from build123d import *

# Parameters (mm, degrees)
SKETCH1_W           = 76.2
SKETCH1_H           = 152.4
BOSS_EXTRUDE1_DEPTH = 3.175
SKETCH2_R           = 4.4196
CUT_EXTRUDE1_DEPTH  = 86.430512699
CUT_EXTRUDE2_DEPTH  = 86.430512699
FILLET1_R           = 12.7


with BuildPart() as part:
    # Sketch1 → Boss-Extrude1 (new, symmetric)
    with BuildSketch(Plane(origin=(0, 0, 0), x_dir=(1, 0, 0), z_dir=(0, 1, 0))):
        Rectangle(SKETCH1_W, SKETCH1_H)
    extrude(amount=BOSS_EXTRUDE1_DEPTH, both=True)

    # Sketch2 → Cut-Extrude1 (cut, through all)
    with BuildSketch(Plane(origin=(0, 3.175, 0), x_dir=(1, 0, 0), z_dir=(0, 1, 0))):
        with Locations(Location((-19.05, 57.15, 0), (0, 0, 270))):
            Circle(SKETCH2_R)
        with Locations(Location((19.05, 57.15, 0), (0, 0, 270))):
            Circle(SKETCH2_R)
        with Locations(Location((19.05, 19.05, 0), (0, 0, 270))):
            Circle(SKETCH2_R)
        with Locations(Location((19.05, -19.05, 0), (0, 0, 270))):
            Circle(SKETCH2_R)
        with Locations(Location((19.05, -57.15, 0), (0, 0, 270))):
            Circle(SKETCH2_R)
        with Locations(Location((-19.05, 19.05, 0), (0, 0, 270))):
            Circle(SKETCH2_R)
        with Locations(Location((-19.05, -19.05, 0), (0, 0, 270))):
            Circle(SKETCH2_R)
        with Locations(Location((-19.05, -57.15, 0), (0, 0, 270))):
            Circle(SKETCH2_R)
    extrude(amount=-CUT_EXTRUDE1_DEPTH, mode=Mode.SUBTRACT)

    # Sketch3 → Cut-Extrude2 (cut, through all)
    with BuildSketch(Plane(origin=(0, 3.175, 0), x_dir=(1, 0, 0), z_dir=(0, 1, 0))):
        Polygon((-38.1, 51.055282861), (-12.955282861, 76.2), (-38.1, 76.2), align=None)
        Polygon((12.955282861, 76.2), (38.1, 76.2), (38.1, 51.055282861), align=None)
    extrude(amount=-CUT_EXTRUDE2_DEPTH, mode=Mode.SUBTRACT)

    # Fillet1
    fillet1_edges = [part.edges().sort_by_distance(p)[0] for p in [
        (-38.1, 0, -51.055282861),
        (-12.955282861, 0, -76.2),
        (38.1, 0, -51.055282861),
        (12.955282861, 0, -76.2),
        (38.1, 0, 76.2),
        (-38.1, 0, 76.2),
    ]]
    fillet(fillet1_edges, radius=FILLET1_R)


solid = part.part
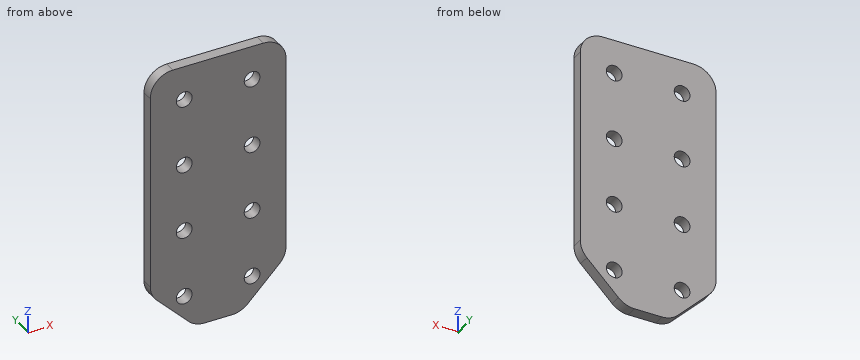
Input: part model. Units: mm. Frame: model coordinates. Give positions to 0.01 mm unless a question says otherwise; leave off trailing zeros. Loops run counter-clockwise (first coordinate to the right, second up) from the corner with the lowest first, then second, coordinate; pieces in that order, holes last. Notation, with made-up numbers: (59.5, 28) -> (76.5, 28) arc R32 ccw to (76.5, 56) -> close; hole circle Ø10 at (66, 57). An arc over 180 degrees is marked (long way). Answer as a JSON object with one key per item and string values. Group by question number.
Item 1: Cut plane B-B, the plane z = -19.05. Return the cut outline in (x, y) (3 decimals).
Item 2: Pin query (flat end, axial travel): P1, Ø14, axis at x = 19.05, z = -19.05, coming from the +Y side (3 decimals). Return the tip coordinate at first contact, or that it passes through.
Item 3: Cut plane C-C, the plane z = -57.15. Return the cut outline in (x, y) (3 decimals), and give its area (3 significant figures).
Item 4: Cut plane A-A, the plane y = -1.75. State how many separate pieces and enclosed holes the cut face has, and give its area (3 significant figures).
Item 5: Line query: probe 1 along X at (y, z) = (0.25, -19.05); probe 2 along Z at (x, y) = (19.5, -2.5); probe 3 along X at (y, z) = (-1, 56.5). Output: solid intervals per line, ascending.
Item 6: Cut plane D-D, the plane x = 28. Return the cut outline in (y, z) (3 decimals), and give its area (4 significant figures).
Checks:
{
 "1": {"outline": "(-38.1, -3.175) -> (-23.47, -3.175) -> (-23.47, 3.175) -> (-38.1, 3.175) -> close; (-14.63, -3.175) -> (14.63, -3.175) -> (14.63, 3.175) -> (-14.63, 3.175) -> close; (23.47, -3.175) -> (38.1, -3.175) -> (38.1, 3.175) -> (23.47, 3.175) -> close"},
 "2": {"P1": "stops at y = 3.175"},
 "3": {"outline": "(-32.005, -3.175) -> (-23.47, -3.175) -> (-23.47, 3.175) -> (-32.005, 3.175) -> close; (-14.63, -3.175) -> (14.63, -3.175) -> (14.63, 3.175) -> (-14.63, 3.175) -> close; (23.47, -3.175) -> (32.005, -3.175) -> (32.005, 3.175) -> (23.47, 3.175) -> close", "area": "294 mm²"},
 "4": {"separate pieces": "1", "enclosed holes": "8", "area": "10,400 mm²"},
 "5": {"probe 1": "x = -38.1 to -23.47, -14.63 to 14.63, 23.47 to 38.1", "probe 2": "z = -69.66 to -61.55, -52.75 to -23.45, -14.65 to 14.65, 23.45 to 52.75, 61.55 to 76.2", "probe 3": "x = -38.1 to -23.42, -14.68 to 14.68, 23.42 to 38.1"},
 "6": {"outline": "(-3.175, -61.155) -> (3.175, -61.155) -> (3.175, 75.931) -> (-3.175, 75.931) -> close", "area": "870.5 mm²"}
}
